Input: part model. Units: mm. Frame: model coordinates. Coordinates: 2 decimals unless noted, no trailing zeros. Order: outer loops, then holes, each group sorted by start corner. A loop starts at its lowest first (then second) coordinate and runs counter-clockwise, first axis right, second up.
from build123d import *

# Parameters (mm, degrees)
BOSS_EXTRUDE1_DEPTH = 6.35
FILLET1_R           = 6.35


with BuildPart() as part:
    # Sketch1 → Boss-Extrude1 (new body)
    with BuildSketch(Plane(origin=(0, 0, 0), x_dir=(1, 0, 0), z_dir=(0, 1, 0))):
        Polygon((-133.35, -146.05), (-146.05, -146.05), (-146.05, 0), (0, 0), (0, -146.05), (-12.7, -146.05), (-12.7, -95.25), (-133.35, -95.25), align=None)
    extrude(amount=BOSS_EXTRUDE1_DEPTH)

    # Fillet1
    fillet1_edges = [part.edges().sort_by_distance(p)[0] for p in [
        (-12.7, 3.175, 95.25),
        (-133.35, 3.175, 95.25),
        (0, 3.175, 146.05),
        (-146.05, 3.175, 0),
        (0, 3.175, 0),
        (-12.7, 3.175, 146.05),
        (-146.05, 3.175, 146.05),
        (-133.35, 3.175, 146.05),
    ]]
    fillet(fillet1_edges, radius=FILLET1_R - 0.0001)  # a hair under: the kernel refuses the full size


solid = part.part
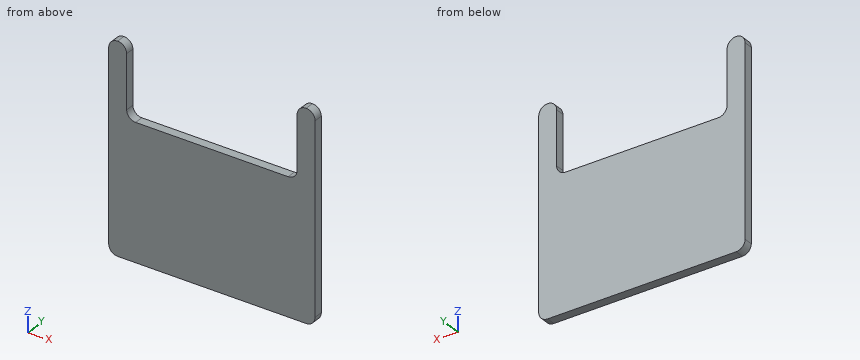
Item 1: Pin query (flat end, axial travel): pin 1 Ø3 at (x, y) = (-25, 1.5) entering from +Z. Return the tip coordinate at first contact, or that it passes through.
Response values:
pin 1: stops at z = 95.25
Item 2: Cut plane C-C on x = -78. Return loops of the section in (y, z).
Response values:
outline: (0, 0) - (6.35, 0) - (6.35, 95.25) - (0, 95.25) - close
Item 3: Cut plane A-A on z = 116. Return loops of the section in (x, y).
Response values:
outline: (-146.05, 0) - (-133.35, 0) - (-133.35, 6.35) - (-146.05, 6.35) - close; (-12.7, 0) - (0, 0) - (0, 6.35) - (-12.7, 6.35) - close
Item 4: Ray query, probe 1 along X at (y, z) = (4.5, 128); probe 2 along Z at (x, y) = (-100, 3.75); probe 3 along Z at (x, y) = (-129.5, 4.25). Return the intervals inside material, ascending.
Response values:
probe 1: x = -146.05 to -133.35, -12.7 to 0
probe 2: z = 0 to 95.25
probe 3: z = 0 to 95.76
